Read the model definition and answer for the solid it produces. Units are mm, in the model's axes. Give positions to 0.01 mm unless a question says otherwise; leave off trailing zeros. Write each loop counter-clockwise with the first axis right and the second up, starting at its lowest first coordinate (ties: lowest second). Pieces come first, ordered by that corner, then holes. Notation, with made-up numbers: (23.5, 11.5) - (47.5, 11.5) arc R11 ccw to (47.5, 29.5) - close; hole circle Ø10 at (-27.5, 34). An arc over 180 degrees is marked (long way). Answer as a JSON object with one key per item and string values. Group by question number.
```python
from build123d import *

# Parameters (mm, degrees)
SKETCH_1_R      = 1.35
SKETCH_1_R_2    = 2.5
EXTRUDE_1_DEPTH = 5


with BuildPart() as part:
    # 草图1 → 凸台-拉伸1 (new body)
    with BuildSketch(Plane.XY):
        with BuildLine():
            Line((-40, 13), (-40, -13))
            ThreePointArc((-40, -13), (-39.414213562, -14.414213562), (-38, -15))
            Line((-38, -15), (42, -15))
            ThreePointArc((42, -15), (57, 0), (42, 15))
            Line((42, 15), (-38, 15))
            ThreePointArc((-38, 15), (-39.414213562, 14.414213562), (-40, 13))
        make_face()
        with Locations((-35, -12)):
            Circle(SKETCH_1_R, mode=Mode.SUBTRACT)
        with Locations((-26.514718626, -8.485281374)):
            Circle(SKETCH_1_R, mode=Mode.SUBTRACT)
        with Locations((-35, 12)):
            Circle(SKETCH_1_R, mode=Mode.SUBTRACT)
        with Locations((-26.514718626, 8.485281374)):
            Circle(SKETCH_1_R, mode=Mode.SUBTRACT)
        with Locations((-23, 0)):
            Circle(SKETCH_1_R, mode=Mode.SUBTRACT)
        with Locations((42, 0)):
            Circle(SKETCH_1_R_2, mode=Mode.SUBTRACT)
    extrude(amount=EXTRUDE_1_DEPTH)


solid = part.part
```
1) Find section C-C, the plane y = 12. Write down the section's boundary in (x, z).
2) Find section B-B, the plane x = -23. Write down the section's boundary in (y, z), and give its area (4 significant figures).
3) Find section A-A, the plane y = 0. Write down the section's boundary in (x, z), and give its area (4 significant figures).
4) Flat-ended cylindrical pins translate along their axes: pin 1 Ø1.6 at (x, y) = (-35, 12) entering from +Z; pin 2 Ø1.5 at (y, z) = (-5.5, 3.5) entering from +X. Find the tip coordinate at first contact, or state that the pin passes through.
5) For a pull along X with two mould halves and no side action, classify faces 1 (the flat face through (3, 15, 2)), 2 (the cylindrical face through (44.31, -0.96, 2.46)), 3 (the cylindrical face through (-39.4, 14.43, 2.46)) as released by +X, released by -X, zero draft, split by the parting line, or undercut.
6) Find the intervals of material crossed by line 1 (X direction, y = 12.5, z = 4.45); line 2 (X direction, y = 8.5, z = 0.3); line 3 (X direction, y = 6.75, z = 0.45), in increasing order. Write a range as [from, to].
7) Find section D-D, the plane z = 2.3. Write down the section's boundary in (x, y).
Values follow:
{
 "1": {"outline": "(-40, 0) - (-36.35, 0) - (-36.35, 5) - (-40, 5) - close; (-33.65, 0) - (51, 0) - (51, 5) - (-33.65, 5) - close"},
 "2": {"outline": "(-15, 0) - (-1.35, 0) - (-1.35, 5) - (-15, 5) - close; (1.35, 0) - (15, 0) - (15, 5) - (1.35, 5) - close", "area": "136.5 mm2"},
 "3": {"outline": "(-40, 0) - (-24.35, 0) - (-24.35, 5) - (-40, 5) - close; (-21.65, 0) - (39.5, 0) - (39.5, 5) - (-21.65, 5) - close; (44.5, 0) - (57, 0) - (57, 5) - (44.5, 5) - close", "area": "446.5 mm2"},
 "4": {"pin 1": "passes through", "pin 2": "stops at x = 56.23"},
 "5": {"face 1": "zero draft", "face 2": "undercut", "face 3": "released by -X"},
 "6": {"line 1": "x = [-40, -36.25], [-33.75, 50.29]", "line 2": "x = [-40, -27.86], [-25.16, 54.36]", "line 3": "x = [-40, 55.4]"},
 "7": {"outline": "(-40, -13) arc R2 ccw to (-38, -15) - (42, -15) arc R15 ccw to (42, 15) - (-38, 15) arc R2 ccw to (-40, 13) - close; hole circle Ø2.7 at (-35, -12); hole circle Ø2.7 at (-35, 12); hole circle Ø2.7 at (-26.51, -8.49); hole circle Ø2.7 at (-26.51, 8.49); hole circle Ø2.7 at (-23, 0); hole circle Ø5 at (42, 0)"}
}
